Source: CAD feature listing. Evaluate the final solid. Frame: model axes, mm. A direction names the side the tool comes from. Give positions to 0.01 mm unless a question says otherwise; leave off trailing zeros. Loops run counter-clockwise (first coordinate to the right, second up) from the corner with the lowest first, then second, coordinate; pieces in that order, holes last. Notation, with made-up numbers: (86.5, 37.5) -> (122.5, 37.5) arc R28 cw to (122.5, 59.5) -> close; hole circle Ø9 at (15.25, -0.75). An arc over 180 degrees is marked (long way). Return JSON: item names as keys, results as strings. Group by question number.
(1) Access query for faces 4 (the face through (-62.9, 36.6, -6.7)), 5 (the face through (-43.433, -36.572, 19.833)), 6 (the face through (-1.449, 36.572, 18.588)), 7 (the face through (30.98, -3.04, -8.62)). Directions: +Z, -Z, +X, -X, +Y, -Y. A direction counts if a zero-diameter tool reaches every point of the face in a straight line with its end or side. Return the directions, or none.
(2) Cut plane D-D on z = 24. Return loops of the section in (x, y), then the cut area to 3 significant figures.
(3) Draft query along X for faces 1 (the face through (0, 0, 18)), 2 (the face through (35, -3, -13.106)), 3 (the face through (31.66, 36.57, -6.7)). Return one class per face: released by +X, released by -X, zero draft, split by the parting line, or undercut.
(4) Cut plane B-B on z = 18. Return loops of the section in (x, y), then the cut area to 3 significant figures.
(5) Ray query, line 1 (X direction, y = -24, z = -10); line 2 (X direction, y = -19, z = -9.5); line 3 (Z direction, x = -75, y = -25.5). Return the intervals inside material, ascending. Write a range as from..to.
(6) Cut plane A-A on y = -1. Return loops of the section in (x, z), then the cut area to 3 significant figures.
(7) Pin query (flat end, axial travel): pin 1 (2 mm diameter, centred on x = 10.5, y = 14, fed in from +Z); pin 2 (12.5 mm diameter, centred on x = -73, y = -6, fed in from -Z); pin 3 (4 mm diameter, centred on y = 2.5, z = 13, fed in from -X). Return the tip coordinate at first contact, or that it passes through.
(8) Cut plane C-C on x = -53. Return loops of the section in (y, z).
```python
from build123d import *

# Parameters (mm, degrees)
F1_DEPTH = 38.1
F2_R     = 5.08


with BuildPart() as f1:
    # F0 (on Front) → F1 (new body, symmetric)
    with BuildSketch(Plane.XZ):
        Polygon((-44.8818020523, 10.0584002212), (-98.5266044736, 10.0584002212), (-98.5266044736, -13.1064001471), (-87.5537991524, -13.1064001471), (-81.152997911, -4.2672003619), (-65.6082034111, -4.2672003619), (-61.6458021104, -13.1064001471), (9.3726003543, -13.1064001471), (13.9445997775, -4.2672003619), (28.8797989488, -4.2672003619), (33.1469997764, -13.1064001471), (42.2910004854, -13.1064001471), (42.2910004854, 6.4007998444), (0, 10.0584002212), (0, 27.4320002645), (-44.8818020523, 27.4320002645), align=None)
    extrude(amount=F1_DEPTH, both=True)

    # F2
    f2_edges = [f1.edges().sort_by_distance(p)[0] for p in [
        (21.412199, 38.1, -4.2672),
        (31.013399, 38.1, -8.6868),
        (37.719, 38.1, -13.1064),
        (42.291, 38.1, -3.3528),
        (21.1455, 38.1, 8.2296),
        (0, 38.1, 18.7452),
        (-22.440901, 38.1, 27.432),
        (-44.881802, 38.1, 18.7452),
        (-71.704203, 38.1, 10.0584),
        (-98.526604, 38.1, -1.524),
        (-93.040202, 38.1, -13.1064),
        (-84.353399, 38.1, -8.6868),
        (-73.380601, 38.1, -4.2672),
        (-63.627003, 38.1, -8.6868),
        (-26.136601, 38.1, -13.1064),
        (11.6586, 38.1, -8.6868),
        (-98.526604, 0, 10.0584),
        (-98.526604, 0, -13.1064),
        (-98.526604, -38.1, -1.524),
        (-44.881802, 0, 27.432),
        (-44.881802, 0, 10.0584),
        (-44.881802, -38.1, 18.7452),
        (0, 0, 10.0584),
        (0, 0, 27.432),
        (0, -38.1, 18.7452),
        (42.291, 0, -13.1064),
        (42.291, 0, 6.4008),
        (42.291, -38.1, -3.3528),
        (-71.704203, -38.1, 10.0584),
        (21.1455, -38.1, 8.2296),
    ]]
    fillet(f2_edges, radius=F2_R)


solid = f1.part
```
Answers:
{
 "1": {"face 4": "-Z, +Y", "face 5": "+Z, -X, -Y", "face 6": "+Z, +X, +Y", "face 7": "-Z, +Y, -Y"},
 "2": {"outline": "(-44.61, -34.67) arc R5.08 ccw to (-39.8, -38.1) -> (-5.08, -38.1) arc R5.08 ccw to (-0.27, -34.67) -> (-0.27, 33.02) arc R4.81 ccw to (-5.08, 37.83) -> (-39.8, 37.83) arc R4.81 ccw to (-44.61, 33.02) -> close", "area": "3,350 mm²"},
 "3": {"face 1": "released by +X", "face 2": "zero draft", "face 3": "undercut"},
 "4": {"outline": "(-44.88, -33.02) arc R5.08 ccw to (-39.8, -38.1) -> (-5.08, -38.1) arc R5.08 ccw to (0, -33.02) -> (0, 33.02) arc R5.08 ccw to (-5.08, 38.1) -> (-39.8, 38.1) arc R5.08 ccw to (-44.88, 33.02) -> close", "area": "3,400 mm²"},
 "5": {"line 1": "-98.13..-85.3, -63.04..10.98, 31.65..41.89", "line 2": "-98.31..-84.94, -63.26..11.24, 31.41..42.07", "line 3": "-4.27..10.06"},
 "6": {"outline": "(-98.53, -8.03) arc R5.08 ccw to (-93.45, -13.11) -> (-87.55, -13.11) -> (-81.15, -4.27) -> (-65.61, -4.27) -> (-61.65, -13.11) -> (9.37, -13.11) -> (13.94, -4.27) -> (28.88, -4.27) -> (33.15, -13.11) -> (37.21, -13.11) arc R5.08 ccw to (42.29, -8.03) -> (42.29, 1.74) arc R5.08 ccw to (37.65, 6.8) -> (4.64, 9.66) arc R5.08 cw to (0, 14.72) -> (0, 22.35) arc R5.08 ccw to (-5.08, 27.43) -> (-39.8, 27.43) arc R5.08 ccw to (-44.88, 22.35) -> (-44.88, 15.14) arc R5.08 cw to (-49.96, 10.06) -> (-93.45, 10.06) arc R5.08 ccw to (-98.53, 4.98) -> close", "area": "3,590 mm²"},
 "7": {"pin 1": "z = 9.24", "pin 2": "z = -4.27", "pin 3": "x = -47.02"},
 "8": {"outline": "(-38.1, -13.11) -> (33.02, -13.11) arc R5.08 ccw to (38.1, -8.03) -> (38.1, 4.98) arc R5.08 ccw to (33.02, 10.06) -> (-33.02, 10.06) arc R5.08 ccw to (-38.1, 4.98) -> close"}
}
